from build123d import *

# Parameters (mm, degrees)
SKETCH1_R           = 5.5
SKETCH1_R_2         = 2.5
BOSS_EXTRUDE1_DEPTH = 20
BOSS_EXTRUDE2_START = -17
SKETCH2_R           = 2.5
BOSS_EXTRUDE2_DEPTH = 2
SKETCH3_R           = 1
CUT_EXTRUDE1_DEPTH  = 2
SKETCH4_R           = 3.5
CUT_EXTRUDE3_DEPTH  = 15


with BuildPart() as part:
    # Sketch1 → Boss-Extrude1 (new body)
    with BuildSketch(Plane.XY):
        Circle(SKETCH1_R)
        Circle(SKETCH1_R_2, mode=Mode.SUBTRACT)
    extrude(amount=BOSS_EXTRUDE1_DEPTH)

    # Sketch2 → Boss-Extrude2 (add)
    with BuildSketch(Plane.XY.offset(20).offset(BOSS_EXTRUDE2_START)):
        Circle(SKETCH2_R)
    extrude(amount=BOSS_EXTRUDE2_DEPTH)

    # Sketch3 → Cut-Extrude1 (cut)
    with BuildSketch(Plane.XY.offset(5)):
        Circle(SKETCH3_R)
    extrude(amount=-CUT_EXTRUDE1_DEPTH, mode=Mode.SUBTRACT)

    # Sketch4 → Cut-Extrude3 (cut)
    with BuildSketch(Plane.XY.offset(20)):
        Circle(SKETCH4_R)
    extrude(amount=-CUT_EXTRUDE3_DEPTH, mode=Mode.SUBTRACT)


solid = part.part
The model under review builds one solid part; all positions refer to its coordinate system, in mm. A direction names the side the tool comes from. Coordinates: 2 decimals unless noted, no trailing zeros. Write each loop counter-clockwise with the first axis right and the second up, starting at its lowest first coordinate (ties: lowest second). Pieces come first, ordered by that corner, then holes. Notation, with made-up numbers: (58, -2) - (107, -2) arc R30 cw to (107, 28) - close; hole circle Ø4 at (-3.5, 9). An arc over 180 degrees is marked (long way). Answer as a JSON object with one key per item and string values. Group by question number.
1. Add section C-C (z = 15.5). Give the boundary of the cut face in (x, y), plus the area to 3 significant figures.
2. Add section D-D (z = 2.25). Give the boundary of the cut face in (x, y), plus the area to 3 significant figures.
3. To check wall thickness, follow probe 1 along Y at (x, z) = (0, 4.1); probe 2 along Z at (x, y) = (-3.25, 0.25); probe 3 along Z at (x, y) = (0.5, -1). State the ranges of each line that lie inside material, in increasing order.
4. Clearance check with flat-ended pins moving along their axes: pin 1 Ø6 at (x, y) = (-2.5, -3) entering from -Z; pin 2 Ø1.5 at (y, z) = (2, 14) entering from +X; pin 3 Ø1.5 at (y, z) = (-2.5, 10) entering from -X; pin 4 Ø5 at (y, z) = (-4, 2.5) entering from +X. State where each tip first meets the part, or that it passes through.
5. Machinability: for faces 4 (the face through (3.233, -1.341, 12.605)), 5 (the face through (0, -1, 4)), 6 (the face through (-0.54, -2.44, 1.48)), which of the approach directions +Z, -Z, +X, -X, +Y, -Y give a long, thin tool a straight path to every point of the face, cutting with its end or side? Answer none if there is none.
6. Add section A-A (y = 0). Give the boundary of the cut face in (x, z).
7. Mouldability with a two-part tool opening along X and no side actions: class faces 1 (the face through (-3, 0, 0)), 2 (the face through (-1.19, -5.37, 9.86)), 3 (the face through (1, -1, 5)) as pulls with the +X half, pulls with the -X half, needs draft (parallel to the pull), parting line crosses it, or undercut.
Findings:
{
 "1": {"outline": "circle Ø11 at (0, 0); hole circle Ø7 at (0, 0)", "area": "56.5 mm²"},
 "2": {"outline": "circle Ø11 at (0, 0); hole circle Ø5 at (0, 0)", "area": "75.4 mm²"},
 "3": {"probe 1": "-5.5 to -1, 1 to 5.5", "probe 2": "0 to 5", "probe 3": "3 to 5"},
 "4": {"pin 1": "z = 0", "pin 2": "x = 5.36", "pin 3": "x = -5.21", "pin 4": "x = 5.29"},
 "5": {"face 4": "+Z", "face 5": "+Z, -Z", "face 6": "-Z"},
 "6": {"outline": "(-5.5, 0) - (-2.5, 0) - (-2.5, 3) - (-1, 3) - (-1, 5) - (-3.5, 5) - (-3.5, 20) - (-5.5, 20) - close; (1, 3) - (2.5, 3) - (2.5, 0) - (5.5, 0) - (5.5, 20) - (3.5, 20) - (3.5, 5) - (1, 5) - close"},
 "7": {"face 1": "needs draft", "face 2": "parting line crosses it", "face 3": "undercut"}
}
